Check sheet for the modelled part. Datum: model origin and axes. Units: mm. A direction names the side the tool comes from. Give positions to 0.01 mm unless a question says otherwise; leave off trailing zeros. Order: outer loops, then holes, each group sorted by start corner. A loop starts at its lowest first (then second) coordinate and runs counter-clockwise, first axis right, second up. Notation, with made-up numbers: M 61.5,69 L 70.5,69 A11 cw 70.5,75 Z; hole C 37.5,47 d7. An arc over 180 degrees is marked long. Answer in a Markdown table with one row per item. Add a question column.
from build123d import *

# Parameters (mm, degrees)
SKETCH1_R           = 62.5
BOSS_EXTRUDE1_DEPTH = 3
SKETCH2_R           = 60
SKETCH2_R_2         = 52.5
BOSS_EXTRUDE2_DEPTH = 10
SKETCH3_R           = 52.5
SKETCH3_R_2         = 50
BOSS_EXTRUDE3_DEPTH = 15
SKETCH4_R           = 50
SKETCH4_R_2         = 42.5
BOSS_EXTRUDE4_DEPTH = 20
SKETCH5_R           = 42.5
CUT_EXTRUDE1_DEPTH  = 4


with BuildPart() as part:
    # Sketch1 → Boss-Extrude1 (new body)
    with BuildSketch(Plane(origin=(0, 0, 0), x_dir=(1, 0, 0), z_dir=(0, 1, 0))):
        Circle(SKETCH1_R)
    extrude(amount=BOSS_EXTRUDE1_DEPTH)

    # Sketch2 → Boss-Extrude2 (add)
    with BuildSketch(Plane(origin=(0, 3, 0), x_dir=(1, 0, 0), z_dir=(0, 1, 0))):
        Circle(SKETCH2_R)
        Circle(SKETCH2_R_2, mode=Mode.SUBTRACT)
    extrude(amount=BOSS_EXTRUDE2_DEPTH)

    # Sketch3 → Boss-Extrude3 (add)
    with BuildSketch(Plane(origin=(0, 3, 0), x_dir=(1, 0, 0), z_dir=(0, 1, 0))):
        Circle(SKETCH3_R)
        Circle(SKETCH3_R_2, mode=Mode.SUBTRACT)
    extrude(amount=BOSS_EXTRUDE3_DEPTH)

    # Sketch4 → Boss-Extrude4 (add)
    with BuildSketch(Plane(origin=(0, 3, 0), x_dir=(1, 0, 0), z_dir=(0, 1, 0))):
        Circle(SKETCH4_R)
        Circle(SKETCH4_R_2, mode=Mode.SUBTRACT)
    extrude(amount=BOSS_EXTRUDE4_DEPTH)

    # Sketch5 → Cut-Extrude1 (cut, through all)
    with BuildSketch(Plane(origin=(0, 3, 0), x_dir=(1, 0, 0), z_dir=(0, 1, 0))):
        Circle(SKETCH5_R)
    extrude(amount=-CUT_EXTRUDE1_DEPTH, mode=Mode.SUBTRACT)


solid = part.part
Q1. Go/stop test with flat-tipped pins: pin 1 (10 mm diameter, centred on x = 12.5, y = 18.5, fed in from +Z); pin 2 (8 mm diameter, centred on y = 16, z = 42, fed in from -X); pin 3 (3 mm diameter, centred on y = 17.5, z = 0, fed in from +X). Record where each tip stops, or that it passes through.
Q2. Cross-section at A-A (x = 0). Record the boundary of the cut face in (y, z).
Q3. Thickness scan on probe 1 along X at (y, z) = (2.45, 0); probe 2 along Z at (x, y) = (0, 13.25); probe 3 along X at (y, z) = (8.75, 15). Record the ranges inside material, lowest first.
Q4. Cross-section at C-C (y = 15.75). Record the boundary of the cut face in (x, z), and give its area (3 significant figures).
Q5. Cross-section at B-B (z = -26.5). Record the boundary of the cut face in (x, y).
Q6. Tool access check on faces 1 (the flat face through (0, 13, 53)), 2 (the cylindrical face through (-62.44, 1.48, -2.75)). Record the directions out of +Z, -Z, +X, -X, +Y, -Y that give a thin tool (end or side, any length) a straight path to the whole face; none if there is none.
Q7. Cross-section at D-D (x = 44). Record the boundary of the cut face in (y, z).
Values follow:
| question | item | result |
|---|---|---|
| 1 | pin 1 | z = 51.96 |
| 1 | pin 2 | x = -45.29 |
| 1 | pin 3 | x = 52.5 |
| 2 | outline | M 0,-62.5 L 3,-62.5 L 3,-60 L 13,-60 L 13,-52.5 L 18,-52.5 L 18,-50 L 23,-50 L 23,-42.5 L 0,-42.5 Z; M 0,42.5 L 23,42.5 L 23,50 L 18,50 L 18,52.5 L 13,52.5 L 13,60 L 3,60 L 3,62.5 L 0,62.5 Z |
| 3 | probe 1 | -62.5 to -42.5, 42.5 to 62.5 |
| 3 | probe 2 | -52.5 to -42.5, 42.5 to 52.5 |
| 3 | probe 3 | -58.09 to -39.76, 39.76 to 58.09 |
| 4 | outline | C 0,0 d105; hole C 0,0 d85 |
| 4 | area | 2,980 mm² |
| 5 | outline | M -56.6,0 L -33.23,0 L -33.23,23 L -42.4,23 L -42.4,18 L -45.32,18 L -45.32,13 L -53.83,13 L -53.83,3 L -56.6,3 Z; M 33.23,0 L 56.6,0 L 56.6,3 L 53.83,3 L 53.83,13 L 45.32,13 L 45.32,18 L 42.4,18 L 42.4,23 L 33.23,23 Z |
| 6 | face 1 | +Y |
| 6 | face 2 | +Y, -Y |
| 7 | outline | M 0,-44.39 L 3,-44.39 L 3,-40.79 L 13,-40.79 L 13,-28.64 L 18,-28.64 L 18,-23.75 L 23,-23.75 L 23,23.75 L 18,23.75 L 18,28.64 L 13,28.64 L 13,40.79 L 3,40.79 L 3,44.39 L 0,44.39 Z |
